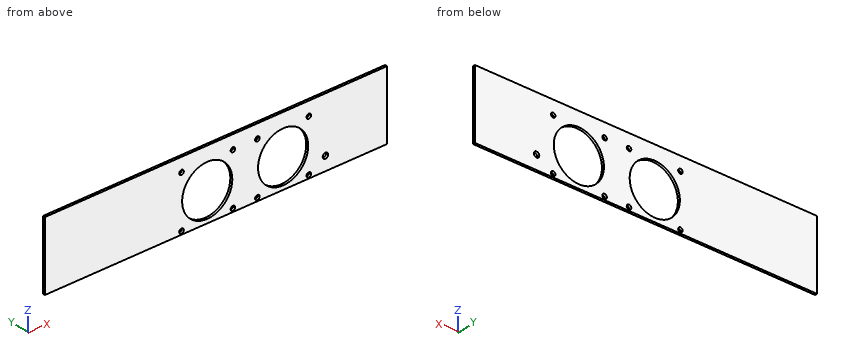
from build123d import *

# Parameters (mm, degrees)
BOSS_EXTRUDE1_DEPTH = 95.25
SKETCH2_R           = 3.175
CUT_EXTRUDE1_DEPTH  = 152.4
SKETCH4_R           = 34.925
SKETCH4_R_2         = 3.81
CUT_EXTRUDE2_DEPTH  = 381
SKETCH5_R           = 3.81
CUT_EXTRUDE3_DEPTH  = 12.7
SKETCH6_W           = 95.25
SKETCH6_H           = 377.825
CUT_EXTRUDE4_DEPTH  = 613.404745654
SKETCH7_W           = 95.25
SKETCH7_H           = 3.175
BOSS_EXTRUDE2_DEPTH = 3.175


with BuildPart() as part:
    # Sketch1 → Boss-Extrude1 (new body)
    with BuildSketch(Plane.XY):
        Polygon((0, 0), (0, 381), (3.175, 381), (3.175, 3.175), (473.075, 3.175), (473.075, 0), align=None)
    extrude(amount=BOSS_EXTRUDE1_DEPTH)

    # Sketch2 → Cut-Extrude1 (cut)
    with BuildSketch(Plane(origin=(0, 3.175, 0), x_dir=(1, 0, 0), z_dir=(0, 1, 0))):
        with Locations(Location((190.119, -4.572, 0), (0, 0, 180))):
            Circle(SKETCH2_R)
        with Locations(Location((190.119, -76.2, 0), (0, 0, 180))):
            Circle(SKETCH2_R)
        with Locations(Location((261.747, -4.572, 0), (0, 0, 180))):
            Circle(SKETCH2_R)
        with Locations(Location((261.747, -76.2, 0), (0, 0, 180))):
            Circle(SKETCH2_R)
        with Locations(Location((295.783, -76.2, 0), (0, 0, 180))):
            Circle(SKETCH2_R)
        with Locations(Location((295.783, -4.572, 0), (0, 0, 180))):
            Circle(SKETCH2_R)
        with Locations(Location((367.411, -76.2, 0), (0, 0, 180))):
            Circle(SKETCH2_R)
        with Locations(Location((367.411, -4.572, 0), (0, 0, 180))):
            Circle(SKETCH2_R)
    extrude(amount=-CUT_EXTRUDE1_DEPTH, mode=Mode.SUBTRACT)

    # Sketch4 → Cut-Extrude2 (cut)
    with BuildSketch(Plane.XZ):
        with Locations((225.933, 40.386)):
            Circle(SKETCH4_R)
        with Locations((331.597, 40.386)):
            Circle(SKETCH4_R)
        with Locations((390.525, 19.05)):
            Circle(SKETCH4_R_2)
    extrude(amount=-CUT_EXTRUDE2_DEPTH, mode=Mode.SUBTRACT)

    # Sketch5 → Cut-Extrude3 (cut)
    with BuildSketch(Plane.ZY):
        with Locations((19.05, 349.25)):
            Circle(SKETCH5_R)
    extrude(amount=-CUT_EXTRUDE3_DEPTH, mode=Mode.SUBTRACT)

    # Sketch6 → Cut-Extrude4 (cut, through all)
    with BuildSketch(Plane(origin=(3.175, 0, 0), x_dir=(0, 0, -1), z_dir=(1, 0, 0))):
        with Locations((-47.625, 192.0875)):
            Rectangle(SKETCH6_W, SKETCH6_H)
    extrude(amount=-CUT_EXTRUDE4_DEPTH, mode=Mode.SUBTRACT)

    # Sketch7 → Boss-Extrude2 (add)
    with BuildSketch(Plane(origin=(473.075, 0, 0), x_dir=(0, 0, -1), z_dir=(1, 0, 0))):
        with Locations((-47.625, 1.5875)):
            Rectangle(SKETCH7_W, SKETCH7_H)
    extrude(amount=BOSS_EXTRUDE2_DEPTH)


solid = part.part
The listing builds one solid part. Answer for the finished solid, in the listing's coordinates (mm). Coordinates: 2 decimals unless noted, no trailing zeros. Loops run counter-clockwise (first coordinate to the right, second up) from the corner with the lowest first, then second, coordinate; pieces in that order, holes last. Notation, with made-up numbers: M -11,-24 L 40,-24 A16 ccw 40,-2 Z; hole C -27.75,-16 d5. An arc over 180 degrees is marked long. Answer in a Markdown table with one row per item.
1) Find section C-C (z = 35.5). Determine the outline of the cut face in (x, y) (3 decimals), then the cut area to 3 significant figures.
Answers below:
| item | result |
|---|---|
| outline | M 0,0 L 191.351,0 L 191.351,3.175 L 0,3.175 Z; M 260.515,0 L 297.015,0 L 297.015,3.175 L 260.515,3.175 Z; M 366.179,0 L 476.25,0 L 476.25,3.175 L 366.179,3.175 Z |
| area | 1,070 mm^2 |
2) Find the intervals of material crossed by probe 1 along X at (y, z) = (2.9, 5); probe 2 along X at (y, z) = (2.35, 15); probe 3 along X at (y, z) = (1.05, 60), in increasing order.
Answers below:
| item | result |
|---|---|
| probe 1 | 0 to 186.97, 193.27 to 258.6, 264.89 to 292.64, 298.93 to 364.26, 370.56 to 476.25 |
| probe 2 | 0 to 201.95, 249.92 to 307.61, 355.58 to 476.25 |
| probe 3 | 0 to 197.04, 254.83 to 302.7, 360.49 to 476.25 |
3) Find section A-A (z = 53). Count the separate pieces of the cut face and the enclosed holes in it, then the cut area to 3 significant figures.
Answers below:
| item | result |
|---|---|
| separate pieces | 3 |
| enclosed holes | 0 |
| area | 1,100 mm^2 |
4) Find section B-B (x = 304). Determine the outline of the cut face in (y, z) (3 decimals), then the cut area to 3 significant figures.
Answers below:
| item | result |
|---|---|
| outline | M 0,0 L 3.175,0 L 3.175,18.981 L 0,18.981 Z; M 0,61.791 L 3.175,61.791 L 3.175,95.25 L 0,95.25 Z |
| area | 166 mm^2 |
